Source: CAD feature listing. Evaluate the final solid. Frame: model axes, mm. Give positions to 0.01 mm unless a question says otherwise; leave off trailing zeros. Order: outer loops, then holes, each group sorted by start corner. A loop starts at its lowest first (then second) coordinate and runs counter-clockwise, first axis right, second up. Notation, with made-up numbers: M -24,-25 L -9,-25 A29 cw -9,-3 Z; hole C 80,24 d5. An arc over 180 degrees is marked long. Use CSV: the item, a comma, the result in double quotes. Start each with the question number.
Item 1: Section query C-C on y = 1.25. Return loops of the section in (x, z), and give its area (3 significant figures).
Item 2: Section query B-B on z = 2.65. Return loops of the section in (x, y), and give its area (3 significant figures).
Item 3: Pull-direction query (Y, two-part tool) for faces 1 (the face through (3, 0, 0)), 2 (the face through (-0.94, 3.01, 1.97)), 3 (the face through (-2.138, -2.317, 1.972)), 4 (the face through (-0.54, 2.44, 1.97)); classes: +Y half, -Y half, draft (parallel to the pull), parting line (faces both ways), or undercut.
Item 4: Section query A-A on x = -0.25. Return loops of the section in (y, z).
Item 5: Ray query, probe 1 along Y at (x, z) = (0, 2.7); probe 2 along X at (y, z) = (-2.25, 3.45); probe 3 along Y at (x, z) = (2.25, 1.8). Return the intervals inside material, ascending. Write a range as from..to.
Item 6: First-contact query: pin 1 (2 mm diameter, centred on y = -2, z = 1.5, fed in from +X); pin 2 (1 mm diameter, centred on y = 2, z = 1.5, fed in from -X). Flat tips, straight axial feed; report the tip coordinate or a pass-through.
Item 7: Section query D-D on y = -2.75. Return loops of the section in (x, z).
Solid Edge part; units mm, degrees
sketch "Sketch1" plane through (0, 0, 0) normal (0, 0, 1) x (1, 0, 0)
  line L0 (2.6952, -2.4472) -> (3.467, 1.1105)
  line L1 (3.467, 1.1105) -> (0.7718, 3.5577)
  line L2 (0.7718, 3.5577) -> (-2.6952, 2.4472)
  line L3 (-2.6952, 2.4472) -> (-3.467, -1.1105)
  line L4 (-3.467, -1.1105) -> (-0.7718, -3.5577)
  line L5 (-0.7718, -3.5577) -> (2.6952, -2.4472)
extrude "Protrusion1" add sketch "Sketch1" along normal blind 4
sketch "Sketch2" plane through (0, 0, 0) normal (0, 0, 1) x (1, 0, 0)
  circle A0 centre (0, 0) radius 2.5
extrude "ExtrudedCutout_1" cut sketch "Sketch2" along normal blind 4
Verdict:
1,outline,"M -2.95,0 L -2.17,0 L -2.17,4 L -2.95,4 Z; M 2.17,0 L 3.31,0 L 3.31,4 L 2.17,4 Z"
1,area,"7.75 mm2"
2,outline,"M -3.47,-1.11 L -0.77,-3.56 L 2.7,-2.45 L 3.47,1.11 L 0.77,3.56 L -2.7,2.45 Z; hole C 0,0 d5"
2,area,"14.8 mm2"
3,face 1,"draft"
3,face 2,"+Y half"
3,face 3,"-Y half"
3,face 4,"undercut"
4,outline,"M -3.39,0 L -2.49,0 L -2.49,4 L -3.39,4 Z; M 2.49,0 L 3.23,0 L 3.23,4 L 2.49,4 Z"
5,probe 1,"-3.31..-2.5, 2.5..3.31"
5,probe 2,"-2.21..-1.09, 1.09..2.74"
5,probe 3,"-2.59..-1.09, 1.09..2.22"
6,pin 1,"x = 3.01"
6,pin 2,"x = -2.9"
7,outline,"M -1.66,0 L 1.75,0 L 1.75,4 L -1.66,4 Z"
